Part model, mm, in its own coordinate system. A direction names the side the tool comes from. Coordinates: 2 decimals unless noted, no trailing zeros. Loops run counter-clockwise (first coordinate to the right, second up) from the corner with the lowest first, then second, coordinate; pieces in that order, holes last. Notation, with made-up numbers: (89.5, 47.25) -> (102.5, 47.25) arc R13 cw to (102.5, 56.25) -> close; hole circle Ø1 at (4, -26.5). An arc over 180 degrees is marked (long way). One line per item, written item: value. Start each with the question number.
from build123d import *

# Parameters (mm, degrees)
F0_W     = 17
F0_H     = 12
F1_DEPTH = 4
F2_R     = 0.75
F3_DEPTH = 25
F5_R     = 6.25
F6_DEPTH = 2.5
F7_R     = 2
F8_R     = 10


with BuildPart() as f1:
    # F0 (on Top) → F1 (new body)
    with BuildSketch(Plane.XY):
        with Locations((0, -6)):
            Rectangle(F0_W, F0_H)
    extrude(amount=F1_DEPTH)

    # F2 (on face) → F3 (cut)
    with BuildSketch(Plane.XY.offset(4)):
        with Locations((-6, -2.5)):
            Circle(F2_R)
        with Locations((6, -2.5)):
            Circle(F2_R)
    extrude(amount=-F3_DEPTH, mode=Mode.SUBTRACT)

    # F5 (on face) → F6 (join)
    with BuildSketch(Plane(origin=(0, -11.8818418781, 4.3246367719), x_dir=(-1, 0, 0), z_dir=(0, 0.9396926208, -0.3420201433))):
        with BuildLine():
            Line((-8.5, -0.3454712368), (8.5, -0.3454712368))
            Line((8.5, -0.3454712368), (8.5, 14.1457582801))
            ThreePointArc((8.5, 14.1457582801), (0, 22.6457582801), (-8.5, 14.1457582801))
            Line((-8.5, 14.1457582801), (-8.5, -0.3454712368))
        make_face()
        with Locations((0, 14.1457582801)):
            Circle(F5_R, mode=Mode.SUBTRACT)
    extrude(amount=F6_DEPTH)

    # F7
    f7_edges = [f1.edges().sort_by_distance(p)[0] for p in [
        (0, -9.339556, 4),
    ]]
    fillet(f7_edges, radius=F7_R)

    # F8
    f8_edges = [f1.edges().sort_by_distance(p)[0] for p in [
        (0, -12, 4),
    ]]
    fillet(f8_edges, radius=F8_R)


solid = f1.part
1) Slice it at B-B (y = -5.25). State how many separate pieces and enclosed holes the cut face has, then the cut area to 3 significant figures.
2) Pin check, flat tips, straight feed: pin 1 Ø1.5 at (y, z) = (-3.5, 20.5) entering from +X; pin 2 Ø3 at (x, z) = (-1, 19) entering from -Y; pin 3 Ø1 at (y, z) = (-4.5, 19) entering from +X; pin 4 Ø0.9 at (x, y) = (6, -2.5) entering from +Z. Stop position of each tip, or through.
3) Probe line 1 (Y direction, x = -6, z = 1.35); line 2 (Z direction, x = 7.5, y = -1.25); line 3 (Z direction, x = -2, y = -3). List the from-to ranges inside material, lowest first. Write a range as from..to.
4) Slice it at A-A (x = 0.75). Give the cut face in (y, z), then the cut area to 3 significant figures.
5) Pull direction Y, two halves, no side cores. Call faces 1 (the cylindrical face through (0.119, -11.844, 3.997)), 2 (the cylindrical face through (5.25, -2.47, 2.03)), 3 (the cylindrical face through (-0.119, -8.106, 4.831)), 4 (the flat face through (0, -3, 4)): +Y half, -Y half, draft (parallel to the pull), parting line (faces both ways), or undercut.
6) Tool access for faces 5 (the cylindrical face through (-6.75, -2.47, 2.03)), 6 (the cylindrical face through (-5.96, -5.24, 18.96)), 7 (the flat face through (-3.7, -6.5, 11.8)): list every direction of +Z, -Z, +X, -X, +Y, -Y with a clear straight run to the whole face (end or side of a thin tool).
7) Slice it at C-C (x = -4.5). Give the cut face in (y, z), then the cut area to 3 significant figures.
8) Slice it at D-D (z = 5). Give the cut face in (x, y), then the cut area to 3 significant figures.
Check sheet entries:
1. separate pieces: 3
1. enclosed holes: 0
1. area: 104 mm^2
2. pin 1: stops at x = 7.89
2. pin 2: passes through
2. pin 3: stops at x = 8.33
2. pin 4: stops at z = 22.85
3. line 1: y = -12..-3.25, -1.75..0
3. line 2: z = 0..4
3. line 3: z = 0..4, 22.45..24.94
4. outline: (-12, 0) -> (0, 0) -> (0, 4) -> (-6.48, 4) arc R2 cw to (-8.36, 6.68) -> (-6.82, 10.93) -> (-9.17, 11.79) -> (-11.4, 5.66) arc R10 ccw to (-12, 2.24) -> close; (-4.92, 23.45) -> (-2.57, 22.59) -> (-1.8, 24.72) -> (-4.15, 25.57) -> close
4. area: 74.9 mm^2
5. face 1: -Y half
5. face 2: undercut
5. face 3: +Y half
5. face 4: draft
6. face 5: -Z
6. face 6: none
6. face 7: +X, -X, +Y
7. outline: (-12, 0) -> (0, 0) -> (0, 4) -> (-6.48, 4) arc R2 cw to (-8.36, 6.68) -> (-6.18, 12.69) -> (-8.53, 13.54) -> (-11.4, 5.66) arc R10 ccw to (-12, 2.24) -> close; (-5.56, 21.69) -> (-3.21, 20.84) -> (-2.23, 23.54) -> (-4.58, 24.39) -> close
7. area: 81.1 mm^2
8. outline: (-8.5, -11.61) -> (8.5, -11.61) -> (8.5, -8.22) -> (-8.5, -8.22) -> close
8. area: 57.7 mm^2
